Model file for the job. Use its own axes, mm. A direction names the side the tool comes from. Coordinates: 2 decimals unless noted, no trailing zeros. Write each loop counter-clockwise with the first axis right and the second up, starting at its lowest first coordinate (ties: lowest second). Pieces come first, ordered by that corner, then holes.
Q1. Band-saw the part on A-A, the plane x = -150. Write the cut outline in (y, z).
Q2. Pull direction Z, two halves, no side cores. Call faces 3 (the flat face through (-152, 25, 0)), 4 (the cylindrical face through (-145.78, 31.33, -123.99)), 5 (the flat face through (-152.1, 25.7, -2)): released by +Z, released by -Z, zero draft, split by the parting line, or undercut.
Q3. Band-saw the part on D-D, the plane z = -110.5. Write the cut outline in (x, y), plus the area to 3 significant figures.
Q4. Band-saw the part on B-B, the plane x = -205. Write the cut outline in (y, z).
Q5. Band-saw the part on C-C, the plane x = -66.5. Write the cut outline in (y, z), plus the area to 3 significant figures.
Q6. Drill centre lines: probe 1 along Z at (x, y) = (-33, 3); probe 2 along Y at (x, z) = (-150, -124); probe 3 along Y at (x, z) = (-162.5, -25.5). Where is each one in solid material? Low to high.
Q7. Pin check, flat tips, straight feed: P1, Ø11.5, axis at x = -150, y = 30, coming from the -Z side; P2, Ø1, axis at x = -169, z = -73.5, coming from the +Y side. Stop position of each tip, or through.
Q8. Which spindle directions (+Z, -Z, +X, -X, +Y, -Y) get a long thin tool onto all of the face, cutting with end or side? Do faces 1 (the flat face through (-152.1, 25.7, -123)), 2 (the flat face through (-300, 1, -62)). Say none if no direction does.
from build123d import *

# Parameters (mm, degrees)
SKETCH1_W           = 300
SKETCH1_H           = 125
BOSS_EXTRUDE1_DEPTH = 50
SHELL1_T            = -2
CUT_EXTRUDE1_DEPTH  = 142
SKETCH3_R           = 4.423757835
CUT_EXTRUDE2_DEPTH  = 132


with BuildPart() as part:
    # Sketch1 → Boss-Extrude1 (new body)
    with BuildSketch(Plane(origin=(0, 0, 0), x_dir=(1, 0, 0), z_dir=(0, 1, 0))):
        with Locations((-150, 62.5)):
            Rectangle(SKETCH1_W, SKETCH1_H)
    extrude(amount=BOSS_EXTRUDE1_DEPTH)

    # Shell1
    shell1_openings = [part.faces().sort_by_distance(p)[0] for p in [
        (-150, 50, -62.5),
        (-300, 25, -62.5),
        (0, 25, -62.5),
    ]]
    offset(amount=SHELL1_T, openings=shell1_openings, kind=Kind.INTERSECTION)

    # Sketch2 → Cut-Extrude1 (cut)
    with BuildSketch(Plane.XY):
        with BuildLine():
            Line((-100, 38), (-50, 38))
            ThreePointArc((-50, 38), (-46, 34), (-50, 30))
            Line((-50, 30), (-100, 30))
            ThreePointArc((-100, 30), (-104, 34), (-100, 38))
        make_face()
    extrude(amount=-CUT_EXTRUDE1_DEPTH, mode=Mode.SUBTRACT)

    # Sketch3 → Cut-Extrude2 (cut)
    with BuildSketch(Plane.XY):
        with Locations((-150, 30)):
            Circle(SKETCH3_R)
    extrude(amount=-CUT_EXTRUDE2_DEPTH, mode=Mode.SUBTRACT)


solid = part.part
Answer sheet:
1. outline: (0, -125) - (25.58, -125) - (25.58, -123) - (2, -123) - (2, -2) - (25.58, -2) - (25.58, 0) - (0, 0) - close; (34.42, -125) - (50, -125) - (50, -123) - (34.42, -123) - close; (34.42, -2) - (50, -2) - (50, 0) - (34.42, 0) - close
2. face 3: released by +Z
2. face 4: zero draft
2. face 5: undercut
3. outline: (-300, 0) - (0, 0) - (0, 2) - (-300, 2) - close
3. area: 600 mm2
4. outline: (0, -125) - (50, -125) - (50, -123) - (2, -123) - (2, -2) - (50, -2) - (50, 0) - (0, 0) - close
5. outline: (0, -125) - (30, -125) - (30, -123) - (2, -123) - (2, -2) - (30, -2) - (30, 0) - (0, 0) - close; (38, -125) - (50, -125) - (50, -123) - (38, -123) - close; (38, -2) - (50, -2) - (50, 0) - (38, 0) - close
5. area: 410 mm2
6. probe 1: z = -125 to -123, -2 to 0
6. probe 2: y = 0 to 25.58, 34.42 to 50
6. probe 3: y = 0 to 2
7. P1: stops at z = -125
7. P2: stops at y = 2
8. face 1: +X, -X, +Y
8. face 2: +Z, -Z, -X, +Y, -Y
